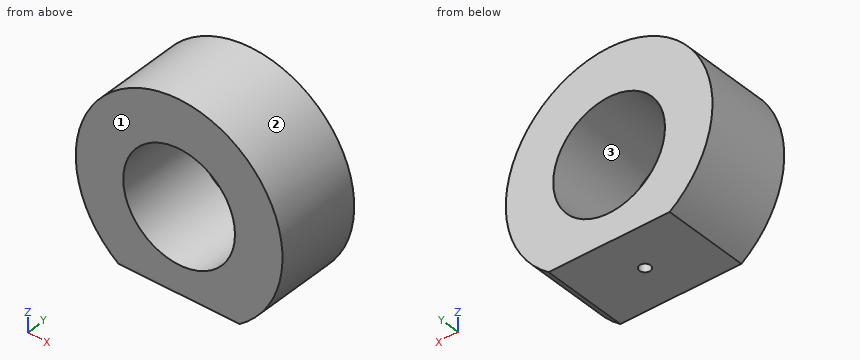
```python
from build123d import *

# Parameters (mm, degrees)
F0_R     = 10
F1_DEPTH = 15.5
F2_R     = 1
F3_DEPTH = 3


with BuildPart() as f1:
    # F0 (on Front) → F1 (new body)
    with BuildSketch(Plane.XZ):
        with BuildLine():
            Line((-10.84, -14.991478), (10.84, -14.991478))
            ThreePointArc((10.84, -14.991478), (0, 18.5), (-10.84, -14.991478))
        make_face()
        Circle(F0_R, mode=Mode.SUBTRACT)
    extrude(amount=F1_DEPTH)

    # F2 (on face) → F3 (cut)
    with BuildSketch(Plane(origin=(0, 0, -14.991478), x_dir=(1, 0, 0), z_dir=(0, 0, -1))):
        with Locations((0, 7.75)):
            Circle(F2_R)
    extrude(amount=-F3_DEPTH, mode=Mode.SUBTRACT)


solid = f1.part
```
Design review of the part built by this model. Coordinates are the model's own, in mm. Face numbers are marked on the shaded views. Coordinates: 2 decimals unless noted, no trailing zeros. Order: outer loops, then holes, each group sorted by start corner. A loop starts at its lowest first (then second) coordinate and runs counter-clockwise, first axis right, second up.
1) Take a section at B-B, the plane x = 0. Give the boundary of the cut face in (y, z), and give its area (3 significant figures).
2) Take a section at C-C, the plane y = -7.75. Give the boundary of the cut face in (x, z).
3) Mouldability with a two-part tool opening along Z and no side actions: class the marked faces 1, 2 and 3 as +Z half, -Z half, draft (parallel to the pull), parting line (faces both ways), or undercut.
4) Take a section at A-A, the plane z = 0. Give the boundary of the cut face in (x, y).
5) Clearance check with a flat-ended pin moving along its axis: pin 1 (2 mm diameter, centred on y = -3.5, z = -2.5, fed in from -X). State where the tip first meets the part, or that it passes through.
6) Wall thickness on line 1 along Y through (x, z) = (0, -14); line 2 along Z through (x, y) = (0, -6.25); line 3 along X through (y, z) = (-12.75, 1): over which ranges is each line inside the solid? List them lowest first.
7) Take a section at D-D, the plane x = -9.5. Give the boundary of the cut face in (y, z).
Returned:
1. outline: (-15.5, -14.99) - (-8.75, -14.99) - (-8.75, -11.99) - (-6.75, -11.99) - (-6.75, -14.99) - (0, -14.99) - (0, -10) - (-15.5, -10) - close; (-15.5, 10) - (0, 10) - (0, 18.5) - (-15.5, 18.5) - close
1. area: 203 mm2
2. outline: (-10.84, -14.99) - (-1, -14.99) - (-1, -11.99) - (1, -11.99) - (1, -14.99) - (10.84, -14.99) arc R18.5 ccw (long way) to start; hole circle Ø20 at (0, 0)
3. face 1: draft
3. face 2: parting line
3. face 3: undercut
4. outline: (-18.5, -15.5) - (-10, -15.5) - (-10, 0) - (-18.5, 0) - close; (10, -15.5) - (18.5, -15.5) - (18.5, 0) - (10, 0) - close
5. pin 1: stops at x = -18.44
6. line 1: y = -15.5 to -8.75, -6.75 to 0
6. line 2: z = -14.99 to -10, 10 to 18.5
6. line 3: x = -18.47 to -9.95, 9.95 to 18.47
7. outline: (-15.5, -14.99) - (0, -14.99) - (0, -3.12) - (-15.5, -3.12) - close; (-15.5, 3.12) - (0, 3.12) - (0, 15.87) - (-15.5, 15.87) - close
